Input: part model. Units: mm. Frame: model coordinates. A direction names the side the tool comes from. Coordinates: 2 decimals unless noted, no trailing zeros. Write each loop counter-clockwise with the first axis right and the second up, starting at its lowest first coordinate (ties: lowest second). Pieces come first, ordered by that corner, then holes. Notation, with made-up numbers: M 44,80.25 L 50,80.25 A31 ccw 50,118.25 Z; hole C 43,46 d8. An arc over 180 degrees is marked long. Write each question's results on one line, items separated by ' | '. Start each with the question number.
1. Section query A-A, the plane x = -25.4. Output: boundary loops of the cut face in (y, z) (3 decimals).
2. Set-up query: faces 5 (the flat face through (-50.8, 18, -32)), 6 (the flat face through (-9, 7.62, -32)), 7 (the flat face through (-31.367, 3.131, -35.131)). Return all of +Z, -Z, +X, -X, +Y, -Y with unobstructed straight access to the full face (end or side cutting, diameter ignored); none if empty.
3. First-contact query: pin 1 (3 mm diameter, centred on x = -9, z = -25.5, fed in from +Y); pin 2 (4 mm diameter, centred on x = -23, z = -29, fed in from -Y); pin 3 (7 mm diameter, centred on y = 19.05, z = -44.45, fed in from -X). Flat tips, straight axial feed; report the tip coordinate or a pass-through.
4. Ray query, probe 1 along X at (y, z) = (13, -47.5); probe 2 along Z at (x, y) = (-3, 19); probe 3 along Y at (x, z) = (-4, -44.45) (3 decimals). Return the intervals inside material, ascending.
5. Pull-direction query (Y, two-part tool) for faces 1 (the flat face through (-19.433, 3.131, -28.369)), 2 (the cylindrical face through (-25.756, 0.724, -62.736)), 3 (the cylindrical face through (-3.19, 19.25, -40.01)), 4 (the flat face through (-3.19, 26.05, -6.26)); classes: +Y half, -Y half, draft (parallel to the pull), parting line (faces both ways), or undercut.
6. Section query C-C, the plane x = -5.5. Output: boundary loops of the cut face in (y, z) (3 decimals).
7. Section query D-D, the plane z = -19.05. Output: boundary loops of the cut face in (x, y) (3 decimals), and give its area (3 significant figures).
8. Section query B-B, the plane y = 8.5. Output: boundary loops of the cut face in (x, z).
```python
from build123d import *

# Parameters (mm, degrees)
SKETCH1_W           = 63.5
SKETCH1_H           = 6.35
BOSS_EXTRUDE1_DEPTH = 50.8
BOSS_EXTRUDE2_DEPTH = 50.8
SKETCH10_W          = 5.842
SKETCH10_H          = 25.629031657
CUT_EXTRUDE1_DEPTH  = 88.854357354
SKETCH11_R          = 4.445
CUT_EXTRUDE2_DEPTH  = 88.854357354
FILLET1_R           = 2.54
SKETCH24_R          = 3.81
CUT_EXTRUDE10_DEPTH = 88.854357354
CUT_EXTRUDE11_DEPTH = 6.35


with BuildPart() as part:
    # Sketch1 → Boss-Extrude1 (new body)
    with BuildSketch(Plane(origin=(0, 0, 0), x_dir=(0, 0, -1), z_dir=(1, 0, 0))):
        with Locations((31.75, 3.175)):
            Rectangle(SKETCH1_W, SKETCH1_H)
    extrude(amount=-BOSS_EXTRUDE1_DEPTH)

    # Sketch2 → Boss-Extrude2 (add)
    with BuildSketch(Plane(origin=(0, 0, 0), x_dir=(0, 0, -1), z_dir=(1, 0, 0))):
        Polygon((0, 6.35), (0, 19.05), (12.7, 33.249031657), (50.8, 33.249031657), (63.5, 19.05), (63.5, 6.35), align=None)
    extrude(amount=-BOSS_EXTRUDE2_DEPTH)

    # Sketch10 → Cut-Extrude1 (cut, through all)
    with BuildSketch(Plane(origin=(0, 0, -63.5), x_dir=(-1, 0, 0), z_dir=(0, 0, -1))):
        with Locations((9.398, 20.434515829)):
            Rectangle(SKETCH10_W, SKETCH10_H)
        with Locations((41.402, 20.434515829)):
            Rectangle(SKETCH10_W, SKETCH10_H)
    extrude(amount=-CUT_EXTRUDE1_DEPTH, mode=Mode.SUBTRACT)

    # Sketch11 → Cut-Extrude2 (cut, through all)
    with BuildSketch(Plane(origin=(0, 0, 0), x_dir=(0, 0, -1), z_dir=(1, 0, 0))):
        with Locations((19.05, 19.05)):
            Circle(SKETCH11_R)
        with Locations((44.45, 19.05)):
            Circle(SKETCH11_R)
    extrude(amount=-CUT_EXTRUDE2_DEPTH, mode=Mode.SUBTRACT)

    # Fillet1
    fillet1_edges = [part.edges().sort_by_distance(p)[0] for p in [
        (0, 0, -31.75),
        (-50.8, 0, -31.75),
        (-25.4, 0, -63.5),
        (-25.4, 0, 0),
    ]]
    fillet(fillet1_edges, radius=FILLET1_R)

    # Sketch24 → Cut-Extrude10 (cut, through all)
    with BuildSketch(Plane.XZ):
        with Locations(Location((-25.4, -31.75, 0), (0, 0, 270))):
            Circle(SKETCH24_R)
    extrude(amount=-CUT_EXTRUDE10_DEPTH, mode=Mode.SUBTRACT)

    # Sketch25 → Cut-Extrude11 (cut)
    with BuildSketch(Plane.XZ):
        Polygon((-29.359468146, -24.892), (-33.318936292, -31.75), (-29.359468146, -38.608), (-21.440531854, -38.608), (-17.481063708, -31.75), (-21.440531854, -24.892), align=None)
    extrude(amount=-CUT_EXTRUDE11_DEPTH, mode=Mode.SUBTRACT)


solid = part.part
```
Answer:
1) outline: M 0,-60.96 A2.54 ccw 2.54,-63.5 L 19.05,-63.5 L 33.249,-50.8 L 33.249,-35.56 L 6.35,-35.56 L 6.35,-38.608 L 0,-38.608 Z; M 0,-24.892 L 6.35,-24.892 L 6.35,-27.94 L 33.249,-27.94 L 33.249,-12.7 L 19.05,0 L 2.54,0 A2.54 ccw 0,-2.54 Z; hole C 19.05,-44.45 d8.89; hole C 19.05,-19.05 d8.89
2) face 5: +Z, -Z, -X, +Y, -Y | face 6: +Z, -Z, +Y | face 7: -Y
3) pin 1: y = 7.62 | pin 2: y = 6.35 | pin 3: through
4) probe 1: -50.8 to -44.32, -38.48 to -12.32, -6.48 to 0 | probe 2: -63.5 to -48.89, -40.01 to -23.49, -14.61 to 0 | probe 3: 0 to 14.605, 23.495 to 33.249
5) face 1: draft | face 2: -Y half | face 3: undercut | face 4: +Y half
6) outline: M 0,-60.96 A2.54 ccw 2.54,-63.5 L 19.05,-63.5 L 33.249,-50.8 L 33.249,-12.7 L 19.05,0 L 2.54,0 A2.54 ccw 0,-2.54 Z; hole C 19.05,-44.45 d8.89; hole C 19.05,-19.05 d8.89
7) outline: M -50.8,2.54 A2.54 ccw -48.26,0 L -2.54,0 A2.54 ccw 0,2.54 L 0,14.605 L -6.477,14.605 L -6.477,7.62 L -12.319,7.62 L -12.319,14.605 L -38.481,14.605 L -38.481,7.62 L -44.323,7.62 L -44.323,14.605 L -50.8,14.605 Z; M -50.8,23.495 L -44.323,23.495 L -44.323,33.249 L -50.8,33.249 Z; M -38.481,23.495 L -12.319,23.495 L -12.319,33.249 L -38.481,33.249 Z; M -6.477,23.495 L 0,23.495 L 0,33.249 L -6.477,33.249 Z | area: 1,040 mm^2
8) outline: M -50.8,-63.5 L -44.32,-63.5 L -44.32,0 L -50.8,0 Z; M -38.48,-63.5 L -12.32,-63.5 L -12.32,0 L -38.48,0 Z; M -6.48,-63.5 L 0,-63.5 L 0,0 L -6.48,0 Z; hole C -25.4,-31.75 d7.62
